Input: part model. Units: mm. Frame: model coordinates. A direction names the side the tool comes from. Coordinates: 2 decimals unless noted, no trailing zeros. Write each loop counter-clockwise with the first axis right and the second up, starting at its lowest first coordinate (ties: lowest second). Pieces come first, ordered by that corner, then holes. Notation, with made-up numbers: (38, -37.5) - (68, -37.5) arc R27 ccw to (68, -11.5) - close; hole circle Ø9 at (65, 60.25). An arc over 180 degrees is marked (long way). Use CSV: the item, a comma, the result in double quotes.
```python
from build123d import *

# Parameters (mm, degrees)
F0_R     = 2.5
F1_DEPTH = 2
F2_R     = 4.5
F3_R     = 1.49999


# Not quite as in the source:
# - a fillet or chamfer is up to 0.001 mm smaller than in the source, because OpenCascade refuses the exact size


with BuildPart() as f1:
    # F0 (on Top) → F1 (new body)
    with BuildSketch(Plane.XY):
        with BuildLine():
            Line((6, -12.5), (12, -12.5))
            Line((12, -12.5), (12, 9.5))
            Line((12, 9.5), (8.25, 9.5))
            Line((8.25, 9.5), (8.25, 4.1809513237))
            ThreePointArc((8.25, 4.1809513237), (9.1721443851, 2.9790199458), (9.5, 1.5))
            ThreePointArc((9.5, 1.5), (8.4748737342, -0.9748737342), (6, -2))
            Line((6, -2), (6, -12.5))
        make_face()
        with BuildLine():
            Line((8.25, 9.5), (12, 9.5))
            Line((12, 9.5), (12, 12.5))
            Line((12, 12.5), (-7, 12.5))
            Line((-7, 12.5), (-7, 11.75))
            ThreePointArc((-7, 11.75), (-5.4090097423, 11.0909902577), (-4.75, 9.5))
            Line((-4.75, 9.5), (-4.75, 4.1809513237))
            ThreePointArc((-4.75, 4.1809513237), (-3.8278556149, 2.9790199458), (-3.5, 1.5))
            ThreePointArc((-3.5, 1.5), (-8.4790199458, -1.6721443851), (-9.25, 4.1809513237))
            Line((-9.25, 4.1809513237), (-9.25, 9.5))
            Line((-9.25, 9.5), (-12, 9.5))
            Line((-12, 9.5), (-12, -7.5))
            Line((-12, -7.5), (-7.25, -7.5))
            ThreePointArc((-7.25, -7.5), (-3, -3.25), (1.25, -7.5))
            ThreePointArc((1.25, -7.5), (0.00520382, -10.50520382), (-3, -11.75))
            Line((-3, -11.75), (-3, -12.5))
            Line((-3, -12.5), (6, -12.5))
            Line((6, -12.5), (6, -2))
            ThreePointArc((6, -2), (2.7111301612, 0.3027802276), (3.75, 4.1809513237))
            Line((3.75, 4.1809513237), (3.75, 9.5))
            ThreePointArc((3.75, 9.5), (6, 11.75), (8.25, 9.5))
        make_face()
        Polygon((-7, 12.5), (12, 12.5), (12, 22.5), (7, 22.5), (-6, 22.5), (-12, 22.5), (-12, 12.5), align=None)
        with BuildLine():
            Line((-12, -12.5), (-3, -12.5))
            Line((-3, -12.5), (-3, -11.75))
            ThreePointArc((-3, -11.75), (-6.00520382, -10.50520382), (-7.25, -7.5))
            Line((-7.25, -7.5), (-12, -7.5))
            Line((-12, -7.5), (-12, -12.5))
        make_face()
        with BuildLine():
            Line((-7, 11.75), (-7, 12.5))
            Line((-7, 12.5), (-12, 12.5))
            Line((-12, 12.5), (-12, 9.5))
            Line((-12, 9.5), (-9.25, 9.5))
            ThreePointArc((-9.25, 9.5), (-8.5909902577, 11.0909902577), (-7, 11.75))
        make_face()
        with BuildLine():
            Line((7, 22.5), (12, 22.5))
            Line((12, 22.5), (12, 43.5))
            Line((12, 43.5), (9.5, 43.5))
            ThreePointArc((9.5, 43.5), (8.767766953, 41.732233047), (7, 41))
            Line((7, 41), (7, 22.5))
        make_face()
        with BuildLine():
            Line((-6, 22.5), (7, 22.5))
            Line((7, 22.5), (7, 41))
            ThreePointArc((7, 41), (5.232233047, 41.732233047), (4.5, 43.5))
            Line((4.5, 43.5), (-6, 43.5))
            Line((-6, 43.5), (-6, 22.5))
        make_face()
        with BuildLine():
            Line((9.5, 43.5), (12, 43.5))
            Line((12, 43.5), (12, 72.5))
            Line((12, 72.5), (0, 72.5))
            Line((0, 72.5), (-16.8, 58.5))
            Line((-16.8, 58.5), (-8.5, 58.5))
            ThreePointArc((-8.5, 58.5), (-6, 61), (-3.5, 58.5))
            ThreePointArc((-3.5, 58.5), (-4.232233047, 56.732233047), (-6, 56))
            Line((-6, 56), (-6, 43.5))
            Line((-6, 43.5), (4.5, 43.5))
            ThreePointArc((4.5, 43.5), (5.232233047, 45.267766953), (7, 46))
            ThreePointArc((7, 46), (8.767766953, 45.267766953), (9.5, 43.5))
        make_face()
        with BuildLine():
            ThreePointArc((9.5, 69.5), (8.767766953, 67.732233047), (7, 67))
            ThreePointArc((7, 67), (5.232233047, 71.267766953), (9.5, 69.5))
        make_face(mode=Mode.SUBTRACT)
        with BuildLine():
            Line((-12, 24), (-12, 22.5))
            Line((-12, 22.5), (-6, 22.5))
            Line((-6, 22.5), (-6, 43.5))
            Line((-6, 43.5), (-6, 56))
            ThreePointArc((-6, 56), (-7.767766953, 56.732233047), (-8.5, 58.5))
            Line((-8.5, 58.5), (-16.8, 58.5))
            Line((-16.8, 58.5), (-18, 57.5))
            Line((-18, 57.5), (-18, 24))
            Line((-18, 24), (-12, 24))
        make_face()
        with Locations((-10, 43.5)):
            Circle(F0_R, mode=Mode.SUBTRACT)
        Polygon((0, 72.5), (12, 72.5), (12, 82.5), align=None)
    extrude(amount=F1_DEPTH)

    # F2
    f2_edges = [f1.edges().sort_by_distance(p)[0] for p in [
        (12, 82.5, 1),
        (-18, 57.5, 1),
        (-12, -12.5, 1),
        (12, -12.5, 1),
        (-18, 24, 1),
    ]]
    fillet(f2_edges, radius=F2_R)

    # F3 (radius 1.5 in the source; OpenCascade refuses exactly that, so slightly less here)
    f3_edges = [f1.edges().sort_by_distance(p)[0] for p in [
        (-12, 24, 1),
    ]]
    fillet(f3_edges, radius=F3_R)


solid = f1.part
```
(1) Reachability of faces 5 (the flat face through (0, -12.5, 1)), 6 (the flat face through (8.25, 7, 1)) from +Z, -Z, +X, -X, +Y, -Y: full face, straight path, thin tool, end or side. Return the list, or none.
Check values:
face 5,"+Z, -Z, +X, -X, -Y"
face 6,"+Z, -Z"
(2) Cut plane A-A on y = 68. Return loops of the section in (x, z).
Check values:
outline,"(-5.4, 0) - (5, 0) - (5, 2) - (-5.4, 2) - close; (9, 0) - (12, 0) - (12, 2) - (9, 2) - close"
(3) Pin query (flat end, axial travel): pin 1 Ø0.6 at (y, z) = (1, 0.5) entering from -X; pin 2 Ø1 at (x, z) = (-14.5, 1) entering from -Y; pin 3 Ø6 at (x, y) = (2.5, 16) entering from -Z; pin 4 Ø1 at (x, z) = (-12, 1) entering from +Y. Return the tip coordinate at first contact, or that it passes through.
Check values:
pin 1,"x = -12"
pin 2,"y = 24.03"
pin 3,"z = 0"
pin 4,"y = 62.92"
(4) Cut plane D-D on x = -15.25. Return loops of the section in (y, z).
Check values:
outline,"(24.35, 0) - (59.79, 0) - (59.79, 2) - (24.35, 2) - close"
(5) Cut plane C-C on z = 1.1. State how many separate pieces and enclosed holes the cut face has, and give its area (3 significant figures).
Check values:
separate pieces,"1"
enclosed holes,"7"
area,"1,950 mm^2"
(6) Draft query along X for faces 1 (the flat face through (0, 33, 0)), 2 (the flat face through (-9.25, 7, 1)), 3 (the cylindrical face through (10.717, -11.147, 1.014)), 4 (the flat face through (-12, 7, 1)). Return one class per face: pulls with the +X half, pulls with the -X half, needs draft (parallel to the pull), parting line crosses it, or undercut.
Check values:
face 1,"needs draft"
face 2,"undercut"
face 3,"pulls with the +X half"
face 4,"pulls with the -X half"
(7) Ray query, probe 1 along Y at (x, z) = (-7.75, 1.4); probe 2 along Y at (x, z) = (-10, 1.6); probe 3 along Y at (x, z) = (-2, 1.8). Return the intervals inside material, ascending. Write a range as from..to.
Check values:
probe 1,"-12.49..-1.92, 11.62..42.41, 44.59..56.71, 60.29..66.04"
probe 2,"-11.74..-0.3, 3.3..41, 46..64.17"
probe 3,"-12.5..-11.63, -3.37..70.83"
(8) Cut plane B-B on x = 0. Return loops of the section in (y, z), and give its area (3 significant figures).
Check values:
outline,"(-12.5, 0) - (-10.51, 0) - (-10.51, 2) - (-12.5, 2) - close; (-4.49, 0) - (72.5, 0) - (72.5, 2) - (-4.49, 2) - close"
area,"158 mm^2"
